```python
from build123d import *

# Parameters (mm, degrees)
BOSS_EXTRUDE4_DEPTH = 15.24
BOSS_EXTRUDE5_DEPTH = 62.865
SKETCH2_11_R        = 10.16
BOSS_EXTRUDE6_DEPTH = 40.64


with BuildPart() as part:
    # Sketch2 → Boss-Extrude4 (new body)
    with BuildSketch(Plane(origin=(0, 0, 0), x_dir=(0, 0, -1), z_dir=(1, 0, 0))):
        with BuildLine():
            Line((10.16, -34.29), (12.7, 31.75))
            ThreePointArc((12.7, 31.75), (0, 44.45), (-12.7, 31.75))
            Line((-12.7, 31.75), (-10.16, -34.29))
            ThreePointArc((-10.16, -34.29), (0, -44.45), (10.16, -34.29))
        make_face()
    extrude(amount=BOSS_EXTRUDE4_DEPTH)

    # Sketch2<9> → Boss-Extrude5 (add)
    with BuildSketch(Plane(origin=(0, 0, 0), x_dir=(0, 0, -1), z_dir=(1, 0, 0))):
        with BuildLine():
            Line((12.662481536, 30.774519941), (12.7, 31.75))
            ThreePointArc((12.7, 31.75), (8.98025611, 40.730256132), (-3e-08, 44.45))
            ThreePointArc((-3e-08, 44.45), (-8.980256132, 40.73025611), (-12.7, 31.75))
            Line((-12.7, 31.75), (-12.662481536, 30.774519941))
            ThreePointArc((-12.662481536, 30.774519941), (0, 19.05), (12.662481536, 30.774519941))
        make_face()
    extrude(amount=BOSS_EXTRUDE5_DEPTH)

    # Sketch2<11> → Boss-Extrude6 (add)
    with BuildSketch(Plane(origin=(0, 0, 0), x_dir=(0, 0, -1), z_dir=(1, 0, 0))):
        with Locations((0, -34.29)):
            Circle(SKETCH2_11_R)
    extrude(amount=BOSS_EXTRUDE6_DEPTH)

    # Mirror1: part across plane


with BuildPart() as part_1:
    add(part.part)
    add(part.part.mirror(Plane(origin=(62.865, 0, 0), x_dir=(0, 0, 1), z_dir=(1, 0, 0))))


solid = part_1.part
```
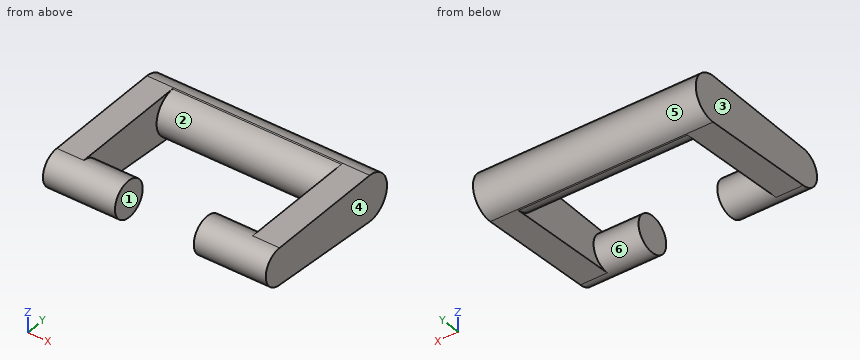
Geometry: final body of the model. Coordinates: model frame, mm. Face numbers are marked on the shaded views. A direction names the side the tool comes from. Coordinates: 2 decimals unless noted, no trailing zeros. Loops run counter-clockwise (first coordinate to the right, second up) from the corner with the lowest first, then second, coordinate; pieces in that order, holes last. Notation, with made-up numbers: (34.5, -39.5) -> (58.5, -39.5) arc R21 ccw to (58.5, -34.5) -> close; hole circle Ø4 at (55, 86). An arc over 180 degrees is marked (long way). Use a Markdown table: item, result. Add a question column.
(1) Section query D-D, the plane y = 23.5. Return loops of the section in (x, z), plus the area to 3 significant figures.
(2) Mould query, pull axis Y, two halves, no side actions, for the marked faces 4, 5 and 6. Classes: pulls with the +Y half, pulls with the -Y half, needs draft (parallel to the pull), parting line crosses it, or undercut.
(3) Section query B-B, the plane x = 30.5. Return loops of the section in (y, z).
(4) Section query C-C, the plane z = 0. Return loops of the section in (x, y).
(5) Section query A-A, the plane y = -32.5. Return loops of the section in (x, z).
(6) Access query for the marked faces 1, 2 and 3. Directions: +Z, -Z, +X, -X, +Y, -Y. A direction counts if a zero-diameter tool reaches every point of the face in a straight line with its end or side. Return the directions, or none.
(7) Line query: line 1 along X through (y, z) = (15.5, -9); line 2 along X through (y, z) = (-26, -1.25); line 3 along Y through (x, z) = (105.5, -8). Output: solid intervals per line, ascending.
(8) Pin query (flat end, axial travel): pin 1 Ø12 at (x, y) = (23.5, 21.5) entering from -Z; pin 2 Ø2 at (x, y) = (33, 33.5) entering from -Z; pin 3 Ø8 at (x, y) = (39, 26.5) entering from -Z. Return the tip coordinate at first contact, or that it passes through.
Answer:
| question | item | result |
|---|---|---|
| 1 | outline | (0, -12.38) -> (15.24, -12.38) -> (15.24, -9.66) -> (110.49, -9.66) -> (110.49, -12.38) -> (125.73, -12.38) -> (125.73, 12.38) -> (110.49, 12.38) -> (110.49, 9.66) -> (15.24, 9.66) -> (15.24, 12.38) -> (0, 12.38) -> close |
| 1 | area | 2,590 mm^2 |
| 2 | face 4 | needs draft |
| 2 | face 5 | pulls with the +Y half |
| 2 | face 6 | undercut |
| 3 | outline | circle Ø20.32 at (-34.29, 0); (30.77, -12.66) -> (31.75, -12.7) arc R12.7 ccw to (31.75, 12.7) -> (30.77, 12.66) arc R12.7 ccw to start |
| 4 | outline | (0, -44.45) -> (40.64, -44.45) -> (40.64, -24.13) -> (15.24, -24.13) -> (15.24, 19.05) -> (110.49, 19.05) -> (110.49, -24.13) -> (85.09, -24.13) -> (85.09, -44.45) -> (125.73, -44.45) -> (125.73, 44.45) -> (0, 44.45) -> close |
| 5 | outline | (0, -10.23) -> (15.24, -10.23) -> (15.24, -10) -> (40.64, -10) -> (40.64, 10) -> (15.24, 10) -> (15.24, 10.23) -> (0, 10.23) -> close; (85.09, -10) -> (110.49, -10) -> (110.49, -10.23) -> (125.73, -10.23) -> (125.73, 10.23) -> (110.49, 10.23) -> (110.49, 10) -> (85.09, 10) -> close |
| 6 | face 1 | +Z, -Z, -Y |
| 6 | face 2 | none |
| 6 | face 3 | +Z, -Z, -X, +Y, -Y |
| 7 | line 1 | x = 0 to 15.24, 110.49 to 125.73 |
| 7 | line 2 | x = 0 to 40.64, 85.09 to 125.73 |
| 7 | line 3 | y = -40.55 to -28.03, 21.89 to 41.61 |
| 8 | pin 1 | stops at z = -11.97 |
| 8 | pin 2 | stops at z = -12.68 |
| 8 | pin 3 | stops at z = -12.64 |
